```python
from build123d import *

# Parameters (mm, degrees)
EXTRUDE_1_DEPTH        = 950
CHAMFER_1_SIZE         = 2
SKETCH_2_R             = 7
CUT_EXTRUDE_1_DEPTH    = 12
PATTERN_LINEAR_1_COUNT = 12
PATTERN_LINEAR_1_PITCH = 80
SKETCH_3_R             = 4.5
CUT_EXTRUDE_2_DEPTH    = 40
PATTERN_LINEAR_2_COUNT = 12
PATTERN_LINEAR_2_PITCH = 80


with BuildPart() as part:
    # 草图1 → 凸台-拉伸1 (new body)
    with BuildSketch(Plane.XY):
        Polygon((-14, 0), (14, 0), (14, 6), (10, 10), (10, 16), (14, 20), (14, 26), (-14, 26), (-14, 20), (-10, 16), (-10, 10), (-14, 6), align=None)
    extrude(amount=EXTRUDE_1_DEPTH)

    # 倒角1
    chamfer_1_edges = [part.edges().sort_by_distance(p)[0] for p in [
        (-14, 26, 475),
        (14, 26, 475),
    ]]
    chamfer(chamfer_1_edges, length=CHAMFER_1_SIZE)

    # 草图2 → 切除-拉伸1 (cut)
    with BuildSketch(Plane(origin=(0, 26, 0), x_dir=(1, 0, 0), z_dir=(0, 1, 0))):
        with Locations(Location((0, -20, 0), (0, 0, 270))):
            Circle(SKETCH_2_R)
    cut_extrude_1 = extrude(amount=-CUT_EXTRUDE_1_DEPTH, mode=Mode.SUBTRACT)

    # 阵列(线性)1: 切除-拉伸1 ×12
    with Locations(*[(0, 0, i * PATTERN_LINEAR_1_PITCH) for i in range(1, PATTERN_LINEAR_1_COUNT)]):
        add(cut_extrude_1, mode=Mode.SUBTRACT)

    # 草图3 → 切除-拉伸2 (cut)
    with BuildSketch(Plane(origin=(0, 26, 0), x_dir=(1, 0, 0), z_dir=(0, 1, 0))):
        with Locations(Location((0, -20, 0), (0, 0, 270))):
            Circle(SKETCH_3_R)
    cut_extrude_2 = extrude(amount=-CUT_EXTRUDE_2_DEPTH, mode=Mode.SUBTRACT)

    # 阵列(线性)2: 切除-拉伸2 ×12
    with Locations(*[(0, 0, i * PATTERN_LINEAR_2_PITCH) for i in range(1, PATTERN_LINEAR_2_COUNT)]):
        add(cut_extrude_2, mode=Mode.SUBTRACT)


solid = part.part
```
The model under review builds one solid part; all positions refer to its coordinate system, in mm. Round coordinates to 2 decimals unless told otherwise and drop trailing zeros. Write each loop counter-clockwise with the first axis right and the second up, starting at its lowest first coordinate (ties: lowest second). Pieces come first, ordered by that corner, then holes.
(1) Wall thickness on L1, parallel to X at y = 20, z = 740; L2, parallel to X at y = 5.25, z = 340; L3, parallel to X at y = 14, z = 551: over which ranges is each line inside the solid? List them lowest first.
(2) We need section A-A on z = 518. Give the boundary of the cut face in (x, y), and give its area (3 significant figures).
(3) We need section B-B on x = 0. Give the number of separate pieces and of enclosed holes in the cut face, and give its area (3 significant figures).
(4) Insertion check: pin 1 (5 mm diameter, centred on y = 13, z = 224, fed in from +X); pin 2 (11.5 mm diameter, centred on x = 0, z = 260, fed in from +Y). Each pin has a flat end and moves straight along its axis. Give the tip position at first contact, or say it passes through.
Findings below:
1. L1: x = -14 to -7, 7 to 14
1. L2: x = -14 to -4.5, 4.5 to 14
1. L3: x = -10 to 10
2. outline: (-14, 0) - (14, 0) - (14, 6) - (10, 10) - (10, 16) - (14, 20) - (14, 24) - (12, 26) - (-12, 26) - (-14, 24) - (-14, 20) - (-10, 16) - (-10, 10) - (-14, 6) - close
2. area: 644 mm2
3. separate pieces: 13
3. enclosed holes: 0
3. area: 21,200 mm2
4. pin 1: stops at x = 10
4. pin 2: stops at y = 14
